Verification items for this drawing (mm, ordinates from the low corner). A direction names the side the tool comes from. Coordinates: 2 decimals unless noted, no trailing zeros. Loops run counter-clockwise (first coordinate to the right, second up) from the corner with the lowest first, then second, coordinate; pieces in that order, holes last. Notation, with made-up numbers: M 45.25,77.5 L 103.25,77.5 A22 ccw 103.25,104.5 Z; hole C 36.5,19.25 d4. An arc over 180 degrees is marked long. Write each question's results on one line, items separated by ' | '. Start each with the question number.
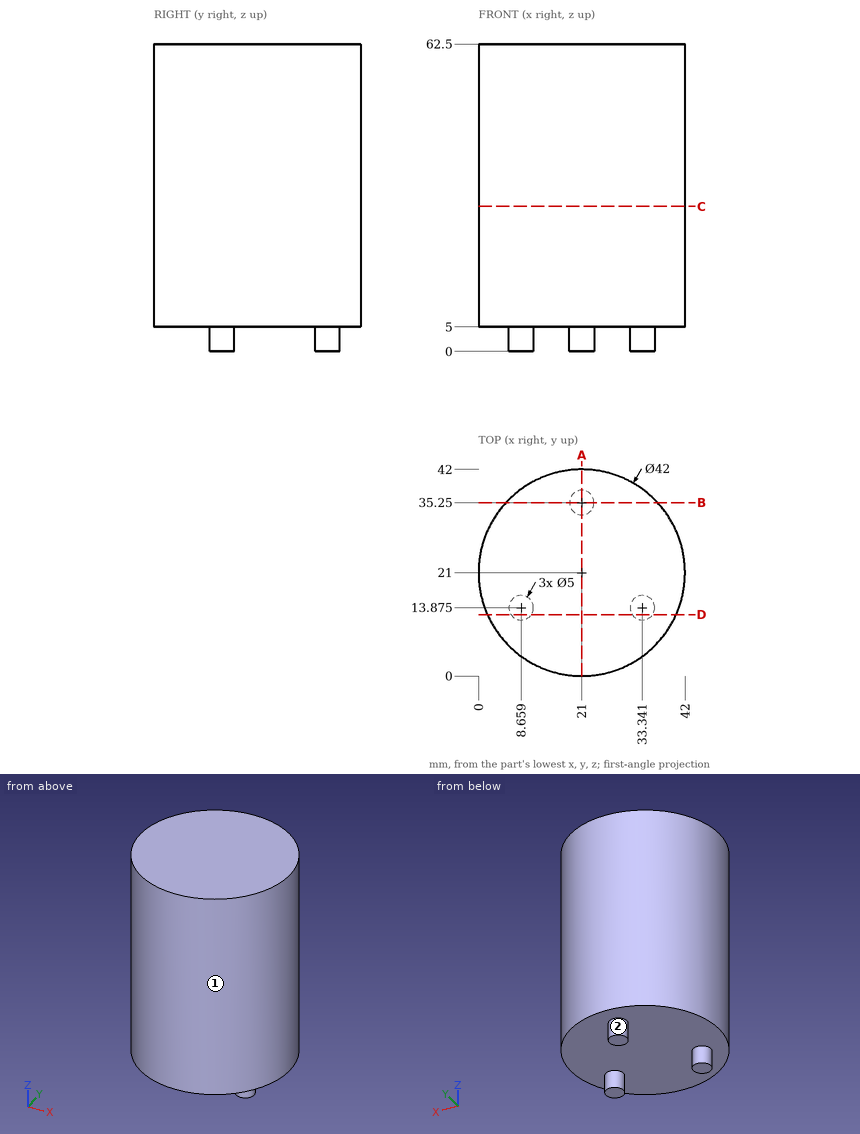
Item 1: Tool access check on the marked faces 1 and 2. Record the directions out of +Z, -Z, +X, -X, +Y, -Y that give a thin tool (end or side, any length) a straight path to the whole face; none if there is none.
Item 2: Depth check by flat-ended pin: P1, Ø6, axis at y = 31.5, z = 22, coming from the -X side (3 decimals); P2, Ø12, axis at y = 28.5, z = 29, coming from the -X side; P3, Ø12.5, axis at x = 23, y = 23, coming from the -Z side. Enter the tip coordinate at first touch or a pass-through.
Item 3: Section check B-B (y = 35.25). Record the cut outline in (x, z) (1 decimal), plus the area to 3 significant figures.
Item 4: Section check C-C (z = 29.5). Record the cut outline in (x, y), plus the area to 3 significant figures.
Item 5: Section check D-D (y = 12.5). Record the cut outline in (x, z), plus the area to 3 significant figures.
Item 6: Section check A-A (x = 21). Record the cut outline in (y, z), plus the area to 3 significant figures.
Item 7: Thickness scan on line 1 (Z direction, x = 10.5, y = 34.5); line 2 (X direction, y = 21.5, z = 25.5); line 3 (Y direction, x = 21, z = 25.5). Record the ranges inside material, lowest first.
Computed values:
1) face 1: +Z, -Z | face 2: -Z
2) P1: stops at x = 1.385 | P2: stops at x = 0.05 | P3: stops at z = 5
3) outline: M 5.6,5 L 18.5,5 L 18.5,0 L 23.5,0 L 23.5,5 L 36.4,5 L 36.4,62.5 L 5.6,62.5 Z | area: 1,800 mm²
4) outline: C 21,21 d42 | area: 1,390 mm²
5) outline: M 1.8,5 L 6.57,5 L 6.57,0 L 10.75,0 L 10.75,5 L 31.25,5 L 31.25,0 L 35.43,0 L 35.43,5 L 40.2,5 L 40.2,62.5 L 1.8,62.5 Z | area: 2,250 mm²
6) outline: M 0,5 L 32.75,5 L 32.75,0 L 37.75,0 L 37.75,5 L 42,5 L 42,62.5 L 0,62.5 Z | area: 2,440 mm²
7) line 1: z = 5 to 62.5 | line 2: x = 0.01 to 41.99 | line 3: y = 0 to 42
